Autodesk Inventor part; units mm, degrees
ref_plane "Work Plane2" through (66.3, 0, 0) normal (1, 0, 0) x (0, 0, -1)
ref_plane "YZ Plane" through (0, 0, 0) normal (1, 0, 0) x (0, 1, 0)
ref_plane "XZ Plane" through (0, 0, 0) normal (0, 1, 0) x (-1, 0, 0)
sketch "Sketch1" plane through (0, 0, 0) normal (0, 0, 1) x (1, 0, 0)
  line L0 (0, 0) -> (132.6, 0)
  line L1 (132.6, 0) -> (132.6, 20)
  line L2 (132.6, 20) -> (0, 20)
  line L3 (0, 20) -> (0, 0)
  line L4 (0, 10) -> (132.6, 10) construction
  line L5 (66.3, 20) -> (66.3, 0) construction
  line L6 (53.45, 9.25) -> (79.15, 9.25)
  line L7 (79.15, 9.25) -> (79.15, 10.75)
  line L8 (79.15, 10.75) -> (53.45, 10.75)
  line L9 (53.45, 10.75) -> (53.45, 9.25)
  line L10 (53.45, 9.25) -> (79.15, 10.75) construction
  line L11 (79.15, 9.25) -> (53.45, 10.75) construction
  line L12 (8, 9.25) -> (25.6, 9.25)
  line L13 (25.6, 9.25) -> (25.6, 10.75)
  line L14 (25.6, 10.75) -> (8, 10.75)
  line L15 (8, 10.75) -> (8, 9.25)
  line L16 (8, 9.25) -> (25.6, 10.75) construction
  line L17 (25.6, 9.25) -> (8, 10.75) construction
  line L18 (107, 9.25) -> (124.6, 9.25)
  line L19 (124.6, 9.25) -> (124.6, 10.75)
  line L20 (124.6, 10.75) -> (107, 10.75)
  line L21 (107, 10.75) -> (107, 9.25)
  line L22 (107, 9.25) -> (124.6, 10.75) construction
  line L23 (124.6, 9.25) -> (107, 10.75) construction
  point P0 (66.3, 10)
  point P1 (16.8, 10)
  point P2 (115.8, 10)
  dimension "d0" = 132.6
  dimension "d1" = 20
  dimension "d2" = 25.7
  dimension "d3" = 1.5
  dimension "d4" = 17.6
  dimension "d5" = 1.5
  dimension "d6" = 49.5
  dimension "d7" = 17.6
  dimension "d8" = 1.5
  dimension "d9" = 49.5
extrude "Extrusion1" add sketch "Sketch1" along normal blind 5.5
ref_plane "Work Plane1" through (0, 10, 0) normal (0, 1, 0) x (1, 0, 0)
ref_plane "Work Plane2" through (66.3, 0, 0) normal (1, 0, 0) x (0, 0, -1)
equation "\"d1\" = midbottomw"
equation "\"d2\" = mmid + toler"
equation "\"d4\" = mlr + toler"
equation "\"d5\" = d3"
equation "\"d7\" = d4"
equation "\"d8\" = d3"
equation "\"thick\" = 0.5"
equation "\"lrlr\" = 19"
equation "\"lrmid\" = 19.9"
equation "\"lrdepth\" = 3.3"
equation "\"mlr\" = 16.6"
equation "\"mmid\" = 24.7"
equation "\"mdepth\" = 4.5"
equation "\"lrltotal\" = 126.6"
equation "\"mltotal\" = 126.6"
equation "\"lrbetween\" = 52.1"
equation "\"mbetween\" = 49.5"
equation "\"toler\" = 1"
equation "\"midbottomw\" = 20"
equation "\"stuckw\" = 6"
equation "\"tight\" = 0.08"
equation "\"sidewallL\" = 132.6"
equation "\"heaterH\" = 117.3"
equation "\"stickL\" = 3.5"
equation "\"wireH\" = 25"
properties part number "mid_bottom"
Verification items for the finished model (mm, model axes). A direction names the side the tool comes from. Give positions to 0.01 mm unless a question says otherwise; leave off trailing zeros. Order: outer loops, then holes, each group sorted by start corner. A loop starts at its lowest first (then second) coordinate and runs counter-clockwise, first axis right, second up. Notation, with made-up numbers: (5.5, 40.25) -> (32.5, 40.25) arc R28 ccw to (32.5, 70.25) -> close; hole circle Ø5 at (-31, -28.75). An arc over 180 degrees is marked (long way). Answer as CSV lines item,"result".
Q1. Access from +Z, -Z, +X, -X, +Y, -Y to the whole of each face (thin tool, end or side, straight path). Record for faces 1 (the flat face through (17, 10.75, 3)), 2 (the flat face through (65, 0, 3)).
Solutions:
face 1,"+Z, -Z"
face 2,"+Z, -Z, +X, -X, -Y"
Q2. Scan lines: probe 1 along X at (y, z) = (10.5, 2.5); probe 2 along Y at (x, z) = (61, 2.05). Record each from-to range of solid material in increasing order.
Solutions:
probe 1,"x = 0 to 8, 25.6 to 53.45, 79.15 to 107, 124.6 to 132.6"
probe 2,"y = 0 to 9.25, 10.75 to 20"
Q3. Release check for a two-part mould opening along X. For faces 3 (the flat face through (116, 9.25, 3)), 4 (the flat face through (67, 20, 3)), 5 (the flat face through (0, 10, 3)) record: +X half, -X half, draft (parallel to the pull), parting line (faces both ways), or undercut.
Solutions:
face 3,"undercut"
face 4,"draft"
face 5,"-X half"
Q4. Sectioned sample at A-A on x = 116.5. Record the cut outline in (y, z), plus the area to 3 significant figures.
Solutions:
outline,"(0, 0) -> (9.25, 0) -> (9.25, 5.5) -> (0, 5.5) -> close; (10.75, 0) -> (20, 0) -> (20, 5.5) -> (10.75, 5.5) -> close"
area,"102 mm²"
Q5. Sectioned sample at B-B on z = 4.25. Record the cut outline in (x, y).
Solutions:
outline,"(0, 0) -> (132.6, 0) -> (132.6, 20) -> (0, 20) -> close; hole (8, 9.25) -> (25.6, 9.25) -> (25.6, 10.75) -> (8, 10.75) -> close; hole (53.45, 9.25) -> (79.15, 9.25) -> (79.15, 10.75) -> (53.45, 10.75) -> close; hole (107, 9.25) -> (124.6, 9.25) -> (124.6, 10.75) -> (107, 10.75) -> close"
